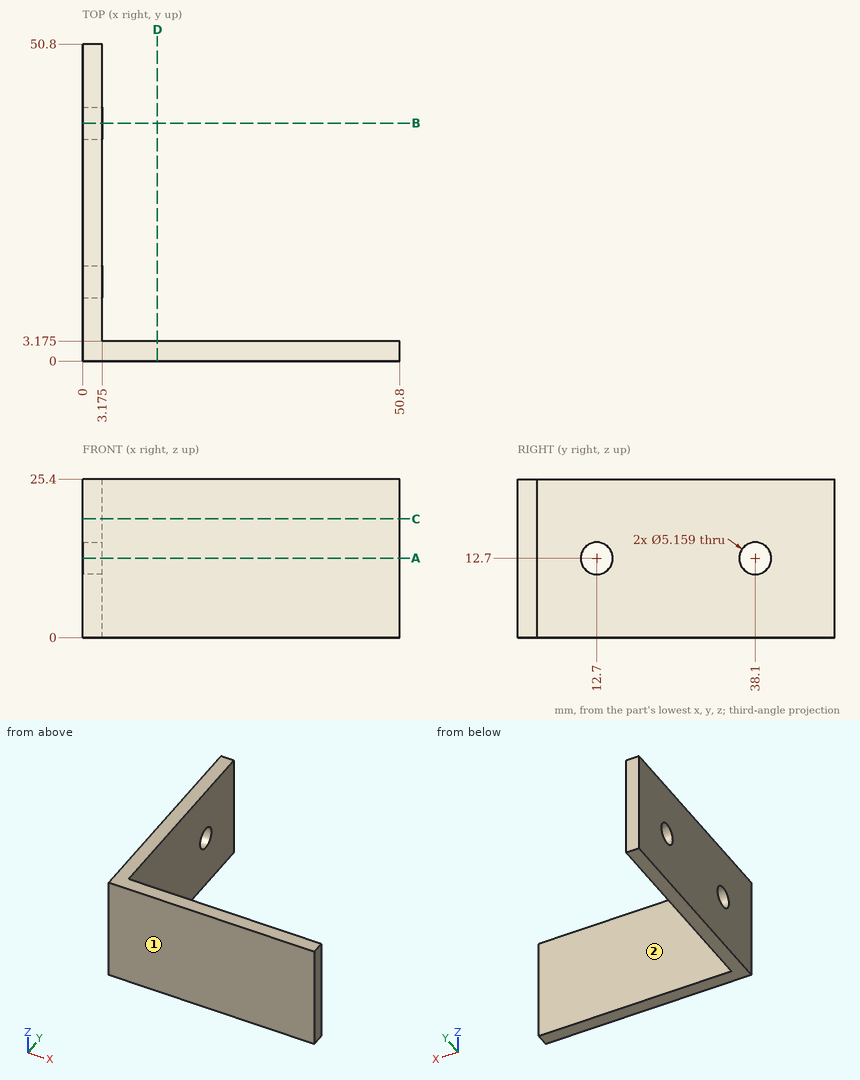
Could you check a few things on this drawing? It's one solid part, dimensions in mm from its lowest x, y, z. A direction names the side the tool comes from. Give positions to 0.01 mm unless a question says otherwise; leave off trailing zeros. Order: outer loops, then holes, each group sorted by start corner. A loop starts at its lowest first (then second) coordinate and runs counter-clockwise, first axis right, second up. Notation, with made-up numbers: (66, 46.5) -> (105, 46.5) arc R19 ccw to (105, 52.5) -> close; hole circle Ø7 at (62, 79.5). An arc over 180 degrees is marked (long way). Answer in a Markdown table with one row per item. Add a question column.
Item 1: Imagine slicing it at B-B (y = 38.1). List the corners of the cut face in (x, z) for me (1 decimal).
Item 2: For the marked faces 1 and 2, which set-ups out of +Z, -Z, +X, -X, +Y, -Y let a thin tool reach every point of the face, with its end or its side?
Item 3: Imagine slicing it at C-C (z = 19). List the corners of the cut face in (x, y) for me (1 decimal).
Item 4: Imagine slicing it at D-D (x = 12). List the corners of the cut face in (y, z) for me (1 decimal).
Item 5: I'm going to push flat-ended pins straight in: P1, Ø5, axis at y = 37.5, z = 13, coming from the +X side (3 decimals); P2, Ø1, axis at x = 39, z = 18.5, coming from the +Y side (3 decimals). Where does each tip first touch, or does it pass through?
Item 6: Imagine slicing it at A-A (z = 12.7). List the corners of the cut face in (x, y) for me (1 decimal), and give its area (3 significant figures).
Item 7: Please list where these lines run through material, in increasing order: probe 1 along Y at (x, z) = (1.1, 12.7); probe 2 along X at (y, z) = (5.5, 7) (1 decimal).
Result:
| question | item | result |
|---|---|---|
| 1 | outline | (0, 0) -> (3.2, 0) -> (3.2, 10.1) -> (0, 10.1) -> close; (0, 15.3) -> (3.2, 15.3) -> (3.2, 25.4) -> (0, 25.4) -> close |
| 2 | face 1 | +Z, -Z, +X, -X, -Y |
| 2 | face 2 | +Z, -Z, +X, +Y |
| 3 | outline | (0, 0) -> (50.8, 0) -> (50.8, 3.2) -> (3.2, 3.2) -> (3.2, 50.8) -> (0, 50.8) -> close |
| 4 | outline | (0, 0) -> (3.2, 0) -> (3.2, 25.4) -> (0, 25.4) -> close |
| 5 | P1 | x = 3.175 |
| 5 | P2 | y = 3.175 |
| 6 | outline | (0, 0) -> (50.8, 0) -> (50.8, 3.2) -> (3.2, 3.2) -> (3.2, 10.1) -> (0, 10.1) -> close; (0, 15.3) -> (3.2, 15.3) -> (3.2, 35.5) -> (0, 35.5) -> close; (0, 40.7) -> (3.2, 40.7) -> (3.2, 50.8) -> (0, 50.8) -> close |
| 6 | area | 280 mm2 |
| 7 | probe 1 | 0 to 10.12, 15.28 to 35.52, 40.68 to 50.8 |
| 7 | probe 2 | 0 to 3.2 |
